Autodesk Inventor part; units mm, degrees
ref_plane "YZ Plane" through (0, 0, 0) normal (1, 0, 0) x (0, 1, 0)
ref_plane "XZ Plane" through (0, 0, 0) normal (0, 1, 0) x (-1, 0, 0)
ref_plane "XY Plane" through (0, 0, 0) normal (0, 0, 1) x (1, 0, 0)
sketch "Sketch1" plane through (0, 0, 0) normal (0, 1, 0) x (-1, 0, 0)
  line L0 (-3, -8) -> (3, -8)
  line L1 (3, -8) -> (3, 8)
  line L2 (3, 8) -> (-3, 8)
  line L3 (-3, 8) -> (-3, -8)
  line L4 (-3, -8) -> (3, 8) construction
  line L5 (3, -8) -> (-3, 8) construction
  point P0 (0, 0)
  dimension "d0" = 6
  dimension "d1" = 16
extrude "Extrusion1" add sketch "Sketch1" along normal blind 10
sketch "Sketch2" plane through (0, 10, 0) normal (0, 1, 0) x (1, 0, 0)
  line L0 (-3, 8) -> (-3, -8)
  line L1 (-3, 0) -> (-1, 0)
  circle A0 centre (-1, 0) radius 1
  point P0 (0, 0)
  dimension "d4" = 2
  dimension "d5" = 2
sketch "Sketch3" plane through (3, 0, -8) normal (0, 0, -1) x (-1, 0, 0)
  line L0 (6, 0) -> (6, 10)
  line L1 (6, 10) -> (10.4832, 2.2349)
  line L2 (6, 10) -> (14.9664, 10) construction
  point P0 (3, 0)
  dimension "d6" = 60
sweep "Sweep1" cut profiles "Sketch2" path "Sketch3" path curves L1
sketch "Sketch5" plane through (3, 0, 8) normal (1, 0, 0) x (0, 0, -1)
  circle A0 centre (3.5, 6.346) radius 2.85
  circle A1 centre (3.5, 6.346) radius 1.55
  circle A2 centre (12.5, 6.346) radius 2.85
  circle A3 centre (12.5, 6.346) radius 1.55
  point P0 (8, 0)
  dimension "d13" = 3.1
  dimension "d14" = 3.1
extrude "Extrusion3" cut sketch "Sketch5" against normal blind 10 contours A1 | A3
properties part number "middleFingerMale"
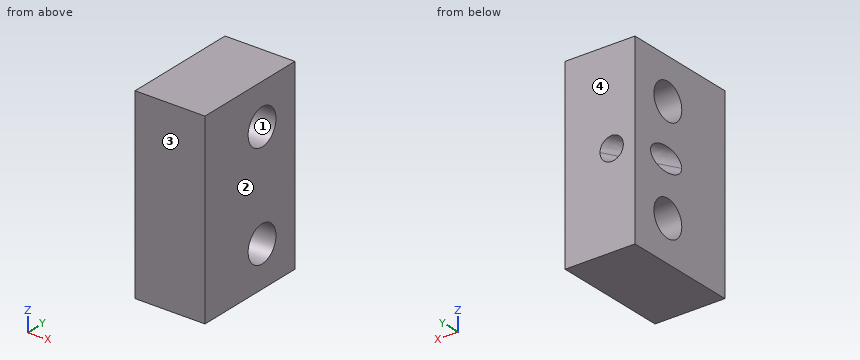
Geometry: final body of the model. Coordinates: model frame, mm. Face numbers are marked on the shaded views. Give positions to 0.01 mm unless a question says otherwise; leave off trailing zeros. Write each loop counter-clockwise with the first axis right and the second up, starting at its lowest first coordinate (ties: lowest second). Pieces come first, ordered by that corner, then holes. Notation, with made-up numbers: (-35, -5.75) -> (24, -5.75) arc R25 ccw to (24, 17.25) -> close; hole circle Ø10 at (50, 63). An arc over 180 degrees is marked (long way). Answer in a Markdown table with one row per item.
(1) Section query B-B on x = 1.25. Return loops of the section in (y, z).
Answers below:
| item | result |
|---|---|
| outline | (0, -8) -> (10, -8) -> (10, 8) -> (0, 8) -> close; hole circle Ø3.1 at (6.35, -4.5); hole circle Ø3.1 at (6.35, 4.5) |
(2) Section query C-C on y = 7. State how many separate pieces and enclosed holes the cut face has, then the cut area to 3 significant figures.
Answers below:
| item | result |
|---|---|
| separate pieces | 3 |
| enclosed holes | 0 |
| area | 60.2 mm^2 |
(3) Ray query, line 1 along Z through (x, y) = (-2.25, 5.5); line 2 along Y through (x, z) = (-1.2, 4.5); line 3 along Z through (x, y) = (0.75, 6.5). Return the intervals inside material, ascending. Write a range as [from, to].
Answers below:
| item | result |
|---|---|
| line 1 | [-8, -5.8], [-3.2, 3.2], [5.8, 8] |
| line 2 | [0, 4.8], [7.9, 10] |
| line 3 | [-8, -6.04], [-2.96, 2.96], [6.04, 8] |
(4) Pin query (flat end, axial travel): pin 1 (3 mm diameter, centred on y = 6.346, z = 4.5, fed in from -X); pin 2 (1 mm diameter, centred on x = -1, z = -1.5, fed in from -Y). Return the tip coordinate at first contact, or that it passes through.
Answers below:
| item | result |
|---|---|
| pin 1 | through |
| pin 2 | y = 0 |
(5) Section query A-A on z = 4.5. Return loops of the section in (x, y).
Answers below:
| item | result |
|---|---|
| outline | (-3, 0) -> (3, 0) -> (3, 4.8) -> (-3, 4.8) -> close; (-3, 7.9) -> (3, 7.9) -> (3, 10) -> (-3, 10) -> close |
(6) Draft query along Y for the marked faces 1, 2, 3 and 4. Return one class per face: +Y half, -Y half, draft (parallel to the pull), parting line (faces both ways), or undercut.
Answers below:
| item | result |
|---|---|
| face 1 | undercut |
| face 2 | draft |
| face 3 | -Y half |
| face 4 | +Y half |
